Read the model definition and answer for the solid it produces. Units are mm, in the model's axes. A direction names the side the tool comes from. Round coordinates to 2 decimals unless told otherwise and drop trailing zeros. Order: outer loops, then holes, each group sorted by start corner. A loop starts at its lowest first (then second) coordinate and runs counter-clockwise, first axis right, second up. Notation, with made-up numbers: (-8, 80.5) - (47, 80.5) arc R21 ccw to (47, 112.5) - close; hole circle Ø9 at (61, 8). An arc over 180 degrees is marked (long way). Answer as a JSON object with one key per item and string values. Group by question number.
Q1. The mould has two halves that part along X. Classify faces 3 (the flat face through (15, -9.525, -146)), 4 (the flat face through (-228.6, -8, -3)), 5 (the flat face through (-3, -8, -203.2)): pulls with the +X half, pulls with the -X half, needs draft (parallel to the pull), parting line crosses it, or undercut.
Q2. A cutting plane is placed at A-A on z = -85. Determine the outline of the cut face in (x, y) (3 decimals), and give its area (3 significant figures).
Q3. A cutting plane is placed at C-C on x = -73.5. Determine the outline of the cut face in (y, z) (3 decimals), and give its area (3 significant figures).
Q4. A tool of negligible diameter and unlimited length cuts with its end or side. For faces 1 (the flat face through (-3, -8, 203.2)), 2 (the flat face through (187.325, -5, -2)), from which of +Z, -Z, +X, -X, +Y, -Y can it reach the whole face along a straight path? Write none if from no direction.
Q5. Consider line 1 (Z direction, x = -61.5, y = -2); line 2 (X direction, y = -3.25, z = -74) (3 decimals); line 3 (Z direction, x = -164, y = -14). Determine where each line is inside the solid, lowest interval first.
Q6. A cutting plane is placed at B-B on y = -6. Determine the outline of the cut face in (x, z) (3 decimals).
```python
from build123d import *

# Parameters (mm, degrees)
F0_W     = 457.2
F0_H     = 406.4
F0_W_2   = 342.9
F0_H_2   = 272.542
F1_DEPTH = 15.875
F2_W     = 374.65
F2_H     = 304.292
F2_W_2   = 342.9
F2_H_2   = 272.542
F3_DEPTH = 9.525


with BuildPart() as f1:
    # F0 (on Front) → F1 (new body)
    with BuildSketch(Plane.XZ):
        Rectangle(F0_W, F0_H)
        Rectangle(F0_W_2, F0_H_2, mode=Mode.SUBTRACT)
    extrude(amount=F1_DEPTH)

    # F2 (on face) → F3 (cut)
    with BuildSketch(Plane(origin=(0, 0, 0), x_dir=(-1, 0, 0), z_dir=(0, 1, 0))):
        Rectangle(F2_W, F2_H)
        Rectangle(F2_W_2, F2_H_2, mode=Mode.SUBTRACT)
    extrude(amount=-F3_DEPTH, mode=Mode.SUBTRACT)


solid = f1.part
```
Result set:
{
 "1": {"face 3": "undercut", "face 4": "pulls with the -X half", "face 5": "needs draft"},
 "2": {"outline": "(-228.6, -15.875) - (-171.45, -15.875) - (-171.45, -9.525) - (-187.325, -9.525) - (-187.325, 0) - (-228.6, 0) - close; (171.45, -15.875) - (228.6, -15.875) - (228.6, 0) - (187.325, 0) - (187.325, -9.525) - (171.45, -9.525) - close", "area": "1,510 mm²"},
 "3": {"outline": "(-15.875, -203.2) - (0, -203.2) - (0, -152.146) - (-9.525, -152.146) - (-9.525, -136.271) - (-15.875, -136.271) - close; (-15.875, 136.271) - (-9.525, 136.271) - (-9.525, 152.146) - (0, 152.146) - (0, 203.2) - (-15.875, 203.2) - close", "area": "1,820 mm²"},
 "4": {"face 1": "+Z, +X, -X, +Y, -Y", "face 2": "+Y"},
 "5": {"line 1": "z = -203.2 to -152.15, 152.15 to 203.2", "line 2": "x = -228.6 to -187.325, 187.325 to 228.6", "line 3": "z = -203.2 to -136.27, 136.27 to 203.2"},
 "6": {"outline": "(-228.6, -203.2) - (228.6, -203.2) - (228.6, 203.2) - (-228.6, 203.2) - close; hole (-187.325, -152.146) - (187.325, -152.146) - (187.325, 152.146) - (-187.325, 152.146) - close"}
}
